Job drawing, mm, ordinate dimensions from the low corner. One solid piece. A direction names the side the tool comes from. Round coordinates to 2 decimals unless told otherwise and drop trailing zeros. Loops run counter-clockwise (first coordinate to the right, second up) from the corner with the lowest first, then second, coordinate; pieces in that order, holes last.
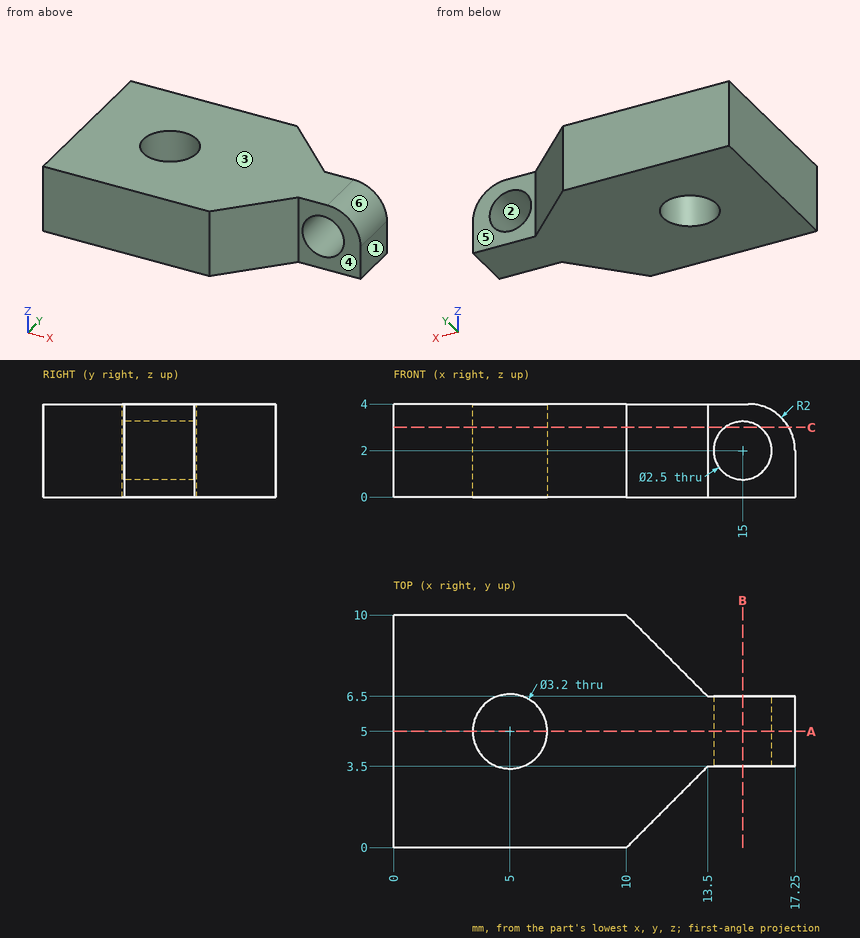
Item 1: Cut at C-C, the plane z = 3. State how many separate pieces and enclosed holes the cut face has, plus the area to 3 significant figures.
Answers follow:
separate pieces: 2
enclosed holes: 1
area: 121 mm2
Item 2: 3-axis set-ups, long thin cutter, end or side, ignore diameter. For the marked faces 4, 5 and 6: which of +Z, -Z, +X, -X, +Y, -Y reach the whole face in a straight line?
Answers follow:
face 4: +Z, -Z, +X, -Y
face 5: +Z, -Z, +X, +Y
face 6: +Z, +X, +Y, -Y
Item 3: Cut at A-A, the plane y = 5. Give the cut face in (x, z), plus the area to 3 significant figures.
Answers follow:
outline: (0, 0) - (3.4, 0) - (3.4, 4) - (0, 4) - close; (6.6, 0) - (17.25, 0) - (17.25, 2) arc R2 ccw to (15.25, 4) - (6.6, 4) - close; hole circle Ø2.5 at (15, 2)
area: 50.4 mm2
Item 4: Two-plate mould, pull along Z, no slides. Class the marked faces 1, 2 and 3: released by +Z, released by -Z, zero draft, split by the parting line, or undercut.
Answers follow:
face 1: zero draft
face 2: undercut
face 3: released by +Z
Item 5: Cut at B-B, the plane x = 15. Give the cut face in (y, z), plus the area to 3 significant figures.
Answers follow:
outline: (3.5, 0) - (6.5, 0) - (6.5, 0.75) - (3.5, 0.75) - close; (3.5, 3.25) - (6.5, 3.25) - (6.5, 4) - (3.5, 4) - close
area: 4.50 mm2
Item 6: Probe line 1 (Y direction, x = 5, z = 2.55); line 2 (Z direction, x = 15, y = 4.7); line 3 (X direction, y = 5.75, z = 0.5). List the from-to ranges inside material, lowest first.
Answers follow:
line 1: y = 0 to 3.4, 6.6 to 10
line 2: z = 0 to 0.75, 3.25 to 4
line 3: x = 0 to 3.59, 6.41 to 17.25
